Source: CAD feature listing. Evaluate the final solid. Frame: model axes, mm. A direction names the side the tool comes from. Give positions to 0.01 mm unless a question says otherwise; leave off trailing zeros. Loops run counter-clockwise (first coordinate to the right, second up) from the corner with the lowest first, then second, coordinate; pieces in that order, holes last. Notation, with made-up numbers: (-18, 24) -> (41, 24) arc R32 cw to (41, 52) -> close; hole circle Ø6 at (40.5, 81.25). An arc over 180 degrees is marked (long way). Put each result on its own line as item: value.
```python
from build123d import *

# Parameters (mm, degrees)
F0_R     = 12.5
F1_DEPTH = 10


with BuildPart() as f1:
    # F0 (on Top) → F1 (new body)
    with BuildSketch(Plane.XY):
        with BuildLine():
            ThreePointArc((0, 17.5), (5.125631, 5.125631), (17.5, 0))
            Line((17.5, 0), (76, 0))
            ThreePointArc((76, 0), (79.535534, 1.464466), (81, 5))
            Line((81, 5), (81, 30))
            ThreePointArc((81, 30), (79.535534, 33.535534), (76, 35))
            Line((76, 35), (17.5, 35))
            ThreePointArc((17.5, 35), (5.125631, 29.874369), (0, 17.5))
        make_face()
        with Locations((17.5, 17.5)):
            Circle(F0_R, mode=Mode.SUBTRACT)
    extrude(amount=F1_DEPTH)

    # F2 (on face) → F3 (revolve, cut)
    with BuildSketch(Plane.XY.offset(10)):
        Polygon((44, 24), (44, 2), (48.5, 2), (48.5, 24), (53, 24), (53, 27), (51.5, 27), (51.5, 32), (44, 32), (44, 27), align=None)
    revolve(axis=Axis((44, 13, 10), (0, 1, 0)), mode=Mode.SUBTRACT)

    # F2 (on face) → F4 (revolve, cut)
    with BuildSketch(Plane.XY.offset(10)):
        Polygon((67, 24), (67, 2), (71.5, 2), (71.5, 24), (76, 24), (76, 27), (74.5, 27), (74.5, 32), (67, 32), (67, 27), align=None)
    revolve(axis=Axis((67, 13, 10), (0, 1, 0)), mode=Mode.SUBTRACT)


solid = f1.part
```
(1) Line query: probe 1 along Y at (x, z) = (17.5, 2); probe 2 along Y at (x, z) = (36, 8.25); probe 3 along X at (y, z) = (14.5, 7.25). Output: solid intervals per line, ascending. Write a range as from..to.
Calculated:
probe 1: y = 0..5, 30..35
probe 2: y = 0..24, 27..35
probe 3: x = 0.26..5.37, 29.63..40.44, 47.56..63.44, 70.56..81
(2) Reachability of faces 4 (the cylindrical face through (44.1, 13.2, 5.5)), 5 (the flat face through (47, 35, 5)) from +Z, -Z, +X, -X, +Y, -Y: full face, straight path, thin tool, end or side. Return the list, or none.
Calculated:
face 4: +Z
face 5: +Z, -Z, +X, -X, +Y
(3) Section B-B on x = 67. Return loops of the section in (y, z), then the cut area to 4 significant figures.
Calculated:
outline: (0, 0) -> (35, 0) -> (35, 10) -> (32, 10) -> (32, 2.5) -> (27, 2.5) -> (27, 1) -> (24, 1) -> (24, 5.5) -> (2, 5.5) -> (2, 10) -> (0, 10) -> close
area: 186.5 mm²
(4) Draft query along Y for faces 1 (the cylindrical face through (80, 33, 5)), 2 (the flat face through (81, 17, 5)), 3 (the cylindrical face through (67, 26, 1)). Return one class per face: released by +Y, released by -Y, zero draft, split by the parting line, or undercut.
Calculated:
face 1: released by +Y
face 2: zero draft
face 3: undercut
(5) Section D-D on x = 22. Return loops of the section in (y, z).
Calculated:
outline: (0, 0) -> (5.84, 0) -> (5.84, 10) -> (0, 10) -> close; (29.16, 0) -> (35, 0) -> (35, 10) -> (29.16, 10) -> close
(6) Section A-A on y = 10.5. Return loops of the section in (x, z), then the cut area to 3 significant figures.
Calculated:
outline: (1.46, 0) -> (7.14, 0) -> (7.14, 10) -> (1.46, 10) -> close; (27.86, 0) -> (81, 0) -> (81, 10) -> (71.5, 10) arc R4.5 cw to (62.5, 10) -> (48.5, 10) arc R4.5 cw to (39.5, 10) -> (27.86, 10) -> close
area: 525 mm²
(7) Section C-C on z = 4.5. Return loops of the section in (x, y), then the cut area to 3 significant figures.
Calculated:
outline: (0, 17.5) arc R17.5 ccw to (17.5, 0) -> (76, 0) arc R5 ccw to (81, 5) -> (81, 30) arc R5 ccw to (76, 35) -> (17.5, 35) arc R17.5 ccw to start; hole circle Ø25 at (17.5, 17.5); hole (36.88, 24) -> (51.12, 24) -> (51.12, 27) -> (49.1, 27) -> (49.1, 32) -> (38.9, 32) -> (38.9, 27) -> (36.88, 27) -> close; hole (59.88, 24) -> (74.12, 24) -> (74.12, 27) -> (72.1, 27) -> (72.1, 32) -> (61.9, 32) -> (61.9, 27) -> (59.88, 27) -> close
area: 2,010 mm²
(8) First-contact query: P1, Ø10, axis at x = 50, y = 26.5, coming from the -Z side; P2, Ø2, axis at x = 14, z = 7.5, coming from the -Y side. Flat tips, straight axial feed; report the tip coordinate or a pass-through.
Calculated:
P1: stops at z = 0
P2: stops at y = 0.18
